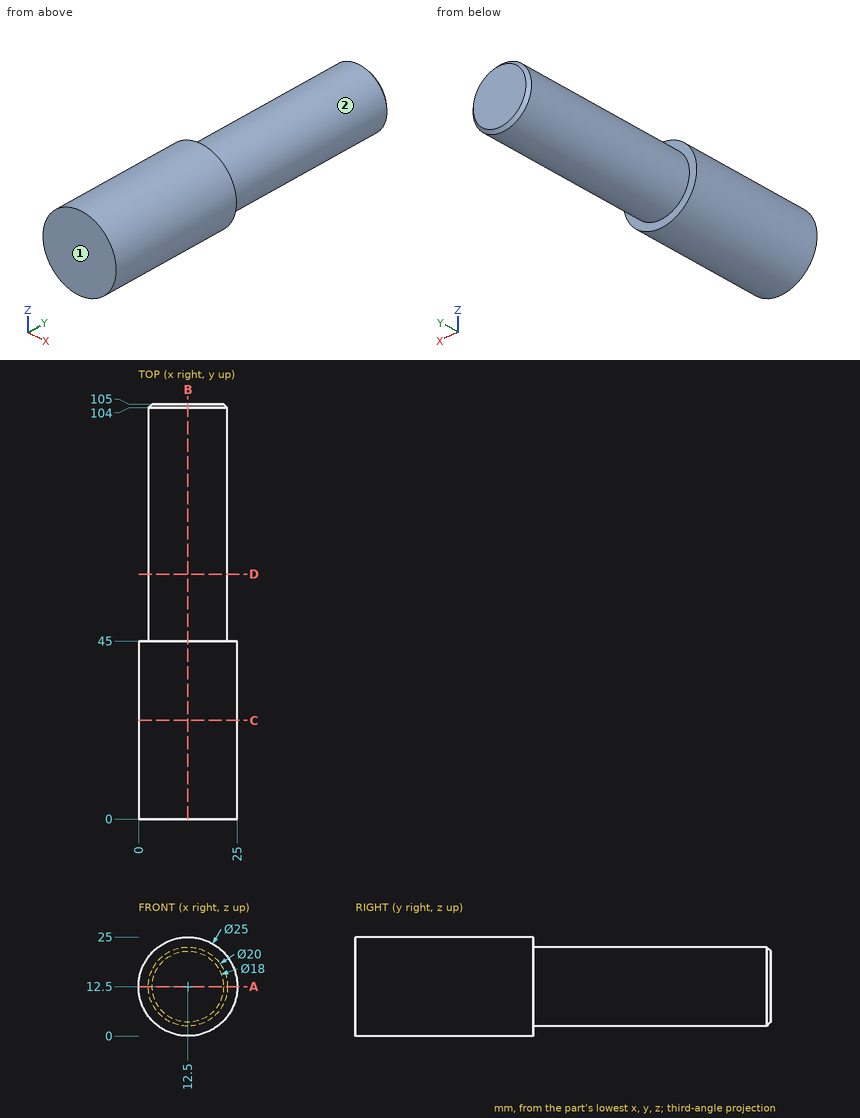
Check sheet for the drawn part. Datum: minimum x, y, z corner. Units: mm. A direction names the side the tool comes from. Give positions to 0.01 mm unless a question says otherwise; leave off trailing zeros. Order: outer loops, then holes, each group sorted by start corner. A loop starts at its lowest first (then second) coordinate and runs counter-clockwise, first axis right, second up. Notation, with made-up numbers: (-5, 84.25) - (1, 84.25) arc R18 cw to (1, 91.25) - close; hole circle Ø5 at (-15.5, 77). An arc over 180 degrees is marked (long way). Write item = value, one per line. Start each with the question number.
1) Access from +Z, -Z, +X, -X, +Y, -Y to the whole of each face (thin tool, end or side, straight path). Record for the marked faces 1 and 2.
2) Section check A-A (z = 12.5). Enter the section's corners in (x, y), then the cut area to 3 significant figures.
3) Gauge pin test, flat ends, axial feed: pin 1 Ø3 at (x, y) = (3, 64.5) entering from -Z; pin 2 Ø1.5 at (x, y) = (22, 13.5) entering from +Z; pin 3 Ø1.5 at (y, z) = (31.5, 19) entering from +X. Record the tip position at first contact, or that the pin passes through.
4) Scan lines: L1, parallel to Y at x = 5, z = 5.75; L2, parallel to X at y = 9.5, z = 12; L3, parallel to X at y = 8.5, z = 5. Record each from-to range of solid material in increasing order.
5) Section check D-D (y = 62). Enter the section's corners in (x, z).
6) Section check C-C (y = 25). Enter the section's corners in (x, z), then the cut area to 3 significant figures.
7) Section check B-B (x = 12.5). Enter the section's corners in (y, z).
Geometry check:
q1.face_1 = +Z, -Z, +X, -X, -Y
q1.face_2 = +Y
q2.outline = (0, 0) - (25, 0) - (25, 45) - (22.5, 45) - (22.5, 104) - (21.5, 105) - (3.5, 105) - (2.5, 104) - (2.5, 45) - (0, 45) - close
q2.area = 2,320 mm2
q3.pin_1 = 6.5
q3.pin_2 = 21.43
q3.pin_3 = 23.6
q4.L1 = 0 to 45
q4.L2 = 0.01 to 24.99
q4.L3 = 2.5 to 22.5
q5.outline = circle Ø20 at (12.5, 12.5)
q6.outline = circle Ø25 at (12.5, 12.5)
q6.area = 491 mm2
q7.outline = (0, 0) - (45, 0) - (45, 2.5) - (104, 2.5) - (105, 3.5) - (105, 21.5) - (104, 22.5) - (45, 22.5) - (45, 25) - (0, 25) - close
